Build history of the part. All positions in model axes, mm. A direction names the side the tool comes from. Give positions to 0.01 mm unless a question says otherwise; leave off trailing zeros. Order: outer loops, then holes, each group sorted by start corner. A loop starts at its lowest first (then second) coordinate and runs counter-clockwise, first axis right, second up. Notation, with made-up numbers: (-23.5, 73) -> (33.5, 73) arc R22 ccw to (33.5, 88) -> close; hole circle Ø9 at (3, -28). An arc over 180 degrees is marked (long way). One line per question, with ' | ' between items. Start each with the question number.
(1) Cut at A-A (y = 22). Give the cut face in (x, z), then the cut area to 3 significant figures.
(2) Pin check, flat tips, straight feed: pin 1 Ø5 at (x, y) = (-14, 23.5) entering from -Z; pin 2 Ø3 at (x, y) = (15, 23) entering from -Z; pin 3 Ø1.8 at (x, z) = (21, -28) entering from -Y. Stop position of each tip, or through.
(3) Cut at C-C (x = 20.5). Give the cut face in (y, z), then the cut area to 3 significant figures.
(4) Which spindle directions (+Z, -Z, +X, -X, +Y, -Y) get a long thin tool onto all of the face, cutting with end or side? Do faces 1 (the face through (0, 4, -21)), 2 (the face through (21.65, 0.99, -29.65)), 3 (the face through (-1, 7, -2)), 4 (the face through (0, 0, -20)), 5 (the face through (0, 15, -2)). Say none if no direction does.
(5) Cut at D-D (z = -22.5). Give the cut face in (x, y), then the cut area to 3 significant figures.
(6) Drill centre lines: L1, parallel to X at y = 22, z = -0.7; L2, parallel to X at y = 0.8, z = -26.88; L3, parallel to Z at x = -1.5, y = 33.5. Where is each one in solid material? Low to high. Write a range as from..to.
(7) Pull direction Z, two halves, no side cores. Call faces 6 (the face through (25, 3, -9)), 7 (the face through (0, 2, -37)), 8 (the face through (-14.26, 3.01, -27.04)), 9 (the face through (19.28, 3.01, -27.15)): +Z half, -Z half, draft (parallel to the pull), parting line (faces both ways), or undercut.
(8) Cut at B-B (z = -26.88). Give the cut face in (x, y), then the cut area to 3 significant figures.
from build123d import *

# Parameters (mm, degrees)
RESSALTO_EXTRUS_O1_DEPTH = 25
CORTE_EXTRUS_O1_START    = -4
ESBO_O2_R                = 3
ESBO_O2_R_2              = 1.25
CORTE_EXTRUS_O1_DEPTH    = 2
ESBO_O2_5_R              = 1.25
CORTE_EXTRUS_O2_DEPTH    = 58.358521599
ESBO_O2_6_R              = 1.25
CORTE_EXTRUS_O3_DEPTH    = 58.358521599
ESBO_O4_R                = 3
ESBO_O4_R_2              = 1.25
CORTE_EXTRUS_O4_DEPTH    = 2
ESBO_O4_4_R              = 1.25
CORTE_EXTRUS_O5_DEPTH    = 58.567351858
CORTE_EXTRUS_O8_START    = -4
CORTE_EXTRUS_O8_DEPTH    = 2
CORTE_EXTRUS_O9_DEPTH    = 58.567351858
FILETE1_R                = 15
FILETE2_R                = 7
FILETE3_R                = 0.25
FILETE4_R                = 3


with BuildPart() as part:
    # Esboço1 → Ressalto-extrusão1 (new, symmetric)
    with BuildSketch(Plane(origin=(0, 0, 0), x_dir=(0, 0, -1), z_dir=(1, 0, 0))):
        Polygon((0, 0), (37, 0), (37, 4), (4, 4), (4, 40), (0, 40), align=None)
    extrude(amount=RESSALTO_EXTRUS_O1_DEPTH, both=True)

    # Esboço2 → Corte-extrusão1 (cut)
    # profile 1 of 2: a face of its own
    with BuildSketch(Plane(origin=(0, 4, 0), x_dir=(1, 0, 0), z_dir=(0, 1, 0)).offset(CORTE_EXTRUS_O1_START)):
        with Locations(Location((20.5, 26.88, 0), (0, 0, 90))):
            Circle(ESBO_O2_R)
        with Locations(Location((20.5, 26.88, 0), (0, 0, 90))):
            Circle(ESBO_O2_R_2, mode=Mode.SUBTRACT)
    # profile 2 of 2: a face of its own
    with BuildSketch(Plane(origin=(0, 4, 0), x_dir=(1, 0, 0), z_dir=(0, 1, 0)).offset(CORTE_EXTRUS_O1_START)):
        with Locations(Location((-15.5, 26.88, 0), (0, 0, 90))):
            Circle(ESBO_O2_R)
        with Locations(Location((-15.5, 26.88, 0), (0, 0, 90))):
            Circle(ESBO_O2_R_2, mode=Mode.SUBTRACT)
    extrude(amount=CORTE_EXTRUS_O1_DEPTH, mode=Mode.SUBTRACT)

    # Esboço2<5> → Corte-extrusão2 (cut, through all)
    with BuildSketch(Plane(origin=(0, 4, 0), x_dir=(1, 0, 0), z_dir=(0, 1, 0))):
        with Locations(Location((-15.5, 26.88, 0), (0, 0, 270))):
            Circle(ESBO_O2_5_R)
    extrude(amount=-CORTE_EXTRUS_O2_DEPTH, mode=Mode.SUBTRACT)

    # Esboço2<6> → Corte-extrusão3 (cut, through all)
    with BuildSketch(Plane(origin=(0, 4, 0), x_dir=(1, 0, 0), z_dir=(0, 1, 0))):
        with Locations(Location((20.5, 26.88, 0), (0, 0, 270))):
            Circle(ESBO_O2_6_R)
    extrude(amount=-CORTE_EXTRUS_O3_DEPTH, mode=Mode.SUBTRACT)

    # Esboço4 → Corte-extrusão4 (cut)
    # profile 1 of 6: a face of its own
    with BuildSketch(Plane(origin=(0, 0, -4), x_dir=(-1, 0, 0), z_dir=(0, 0, -1))):
        with Locations(Location((14, 22, 0), (0, 0, 90))):
            Circle(ESBO_O4_R)
        with Locations(Location((14, 22, 0), (0, 0, 90))):
            Circle(ESBO_O4_R_2, mode=Mode.SUBTRACT)
    # profile 2 of 6: a face of its own
    with BuildSketch(Plane(origin=(0, 0, -4), x_dir=(-1, 0, 0), z_dir=(0, 0, -1))):
        with Locations(Location((-14, 22, 0), (0, 0, 90))):
            Circle(ESBO_O4_R)
        with Locations(Location((-14, 22, 0), (0, 0, 90))):
            Circle(ESBO_O4_R_2, mode=Mode.SUBTRACT)
    # profile 3 of 6: a face of its own
    with BuildSketch(Plane(origin=(0, 0, -4), x_dir=(-1, 0, 0), z_dir=(0, 0, -1))):
        with BuildLine():
            ThreePointArc((3, 8), (2.121320344, 10.121320344), (0, 11))
            Line((0, 11), (0, 9.25))
            ThreePointArc((0, 9.25), (0.883883476, 8.883883476), (1.25, 8))
            ThreePointArc((1.25, 8), (0.883883476, 7.116116524), (0, 6.75))
            Line((0, 6.75), (0, 5))
            ThreePointArc((0, 5), (2.121320344, 5.878679656), (3, 8))
        make_face()
    # profile 4 of 6: a face of its own
    with BuildSketch(Plane(origin=(0, 0, -4), x_dir=(-1, 0, 0), z_dir=(0, 0, -1))):
        with BuildLine():
            Line((0, 9.25), (0, 11))
            ThreePointArc((0, 11), (-3, 8), (0, 5))
            Line((0, 5), (0, 6.75))
            ThreePointArc((0, 6.75), (-1.25, 8), (0, 9.25))
        make_face()
    # profile 5 of 6: a face of its own
    with BuildSketch(Plane(origin=(0, 0, -4), x_dir=(-1, 0, 0), z_dir=(0, 0, -1))):
        with BuildLine():
            ThreePointArc((3, 8), (2.121320344, 10.121320344), (0, 11))
            Line((0, 11), (0, 9.25))
            ThreePointArc((0, 9.25), (0.883883476, 8.883883476), (1.25, 8))
            ThreePointArc((1.25, 8), (0.883883476, 7.116116524), (0, 6.75))
            Line((0, 6.75), (0, 5))
            ThreePointArc((0, 5), (2.121320344, 5.878679656), (3, 8))
        make_face()
    # profile 6 of 6: a face of its own
    with BuildSketch(Plane(origin=(0, 0, -4), x_dir=(-1, 0, 0), z_dir=(0, 0, -1))):
        with BuildLine():
            Line((0, 9.25), (0, 11))
            ThreePointArc((0, 11), (-3, 8), (0, 5))
            Line((0, 5), (0, 6.75))
            ThreePointArc((0, 6.75), (-1.25, 8), (0, 9.25))
        make_face()
    extrude(amount=-CORTE_EXTRUS_O4_DEPTH, mode=Mode.SUBTRACT)

    # Esboço4<4> → Corte-extrusão5 (cut, through all)
    with BuildSketch(Plane(origin=(0, 0, -4), x_dir=(-1, 0, 0), z_dir=(0, 0, -1))):
        with Locations(Location((-14, 22, 0), (0, 0, 90))):
            Circle(ESBO_O4_4_R)
        with Locations(Location((14, 22, 0), (0, 0, 90))):
            Circle(ESBO_O4_4_R)
        with BuildLine():
            ThreePointArc((1.25, 8), (0.883883476, 8.883883476), (0, 9.25))
            Line((0, 9.25), (0, 6.75))
            ThreePointArc((0, 6.75), (0.883883476, 7.116116524), (1.25, 8))
        make_face()
        with BuildLine():
            Line((0, 6.75), (0, 9.25))
            ThreePointArc((0, 9.25), (-1.25, 8), (0, 6.75))
        make_face()
    extrude(amount=-CORTE_EXTRUS_O5_DEPTH, mode=Mode.SUBTRACT)

    # Esboço4<11> → Corte-extrusão8 (cut)
    with BuildSketch(Plane(origin=(0, 0, -4), x_dir=(-1, 0, 0), z_dir=(0, 0, -1)).offset(CORTE_EXTRUS_O8_START)):
        with BuildLine():
            ThreePointArc((3, 16.65), (2.121320344, 18.771320344), (0, 19.65))
            Line((0, 19.65), (0, 17.9))
            ThreePointArc((0, 17.9), (0.883883476, 17.533883476), (1.25, 16.65))
            ThreePointArc((1.25, 16.65), (0.883883476, 15.766116524), (0, 15.4))
            Line((0, 15.4), (0, 13.65))
            ThreePointArc((0, 13.65), (2.121320344, 14.528679656), (3, 16.65))
        make_face()
        with BuildLine():
            Line((0, 17.9), (0, 19.65))
            ThreePointArc((0, 19.65), (-3, 16.65), (0, 13.65))
            Line((0, 13.65), (0, 15.4))
            ThreePointArc((0, 15.4), (-1.25, 16.65), (0, 17.9))
        make_face()
        with BuildLine():
            ThreePointArc((3, 35), (2.121320344, 37.121320344), (0, 38))
            Line((0, 38), (0, 36.25))
            ThreePointArc((0, 36.25), (0.883883476, 35.883883476), (1.25, 35))
            ThreePointArc((1.25, 35), (0.883883476, 34.116116524), (0, 33.75))
            Line((0, 33.75), (0, 32))
            ThreePointArc((0, 32), (2.121320344, 32.878679656), (3, 35))
        make_face()
        with BuildLine():
            Line((0, 36.25), (0, 38))
            ThreePointArc((0, 38), (-3, 35), (0, 32))
            Line((0, 32), (0, 33.75))
            ThreePointArc((0, 33.75), (-1.25, 35), (0, 36.25))
        make_face()
    extrude(amount=CORTE_EXTRUS_O8_DEPTH, mode=Mode.SUBTRACT)

    # Esboço4<12> → Corte-extrusão9 (cut, through all)
    with BuildSketch(Plane(origin=(0, 0, -4), x_dir=(-1, 0, 0), z_dir=(0, 0, -1))):
        with BuildLine():
            ThreePointArc((1.25, 35), (0.883883476, 35.883883476), (0, 36.25))
            Line((0, 36.25), (0, 33.75))
            ThreePointArc((0, 33.75), (0.883883476, 34.116116524), (1.25, 35))
        make_face()
        with BuildLine():
            Line((0, 33.75), (0, 36.25))
            ThreePointArc((0, 36.25), (-1.25, 35), (0, 33.75))
        make_face()
        with BuildLine():
            ThreePointArc((1.25, 16.65), (0.883883476, 17.533883476), (0, 17.9))
            Line((0, 17.9), (0, 15.4))
            ThreePointArc((0, 15.4), (0.883883476, 15.766116524), (1.25, 16.65))
        make_face()
        with BuildLine():
            Line((0, 15.4), (0, 17.9))
            ThreePointArc((0, 17.9), (-1.25, 16.65), (0, 15.4))
        make_face()
    extrude(amount=-CORTE_EXTRUS_O9_DEPTH, mode=Mode.SUBTRACT)

    # Filete1
    filete1_edges = [part.edges().sort_by_distance(p)[0] for p in [
        (25, 40, -2),
        (-25, 40, -2),
    ]]
    fillet(filete1_edges, radius=FILETE1_R)

    # Filete2
    filete2_edges = [part.edges().sort_by_distance(p)[0] for p in [
        (25, 2, -37),
        (-25, 2, -37),
    ]]
    fillet(filete2_edges, radius=FILETE2_R)

    # Filete3
    filete3_edges = [part.edges().sort_by_distance(p)[0] for p in [
        (0, 4, -4),
    ]]
    fillet(filete3_edges, radius=FILETE3_R)

    # Filete4
    filete4_edges = [part.edges().sort_by_distance(p)[0] for p in [
        (0, 0, 0),
    ]]
    fillet(filete4_edges, radius=FILETE4_R)


solid = part.part
Result set:
1) outline: (-25, -4) -> (-17, -4) -> (-17, -2) -> (-15.25, -2) -> (-15.25, 0) -> (-25, 0) -> close; (-12.75, -2) -> (-11, -2) -> (-11, -4) -> (11, -4) -> (11, -2) -> (12.75, -2) -> (12.75, 0) -> (-12.75, 0) -> close; (15.25, -2) -> (17, -2) -> (17, -4) -> (25, -4) -> (25, 0) -> (15.25, 0) -> close | area: 166 mm2
2) pin 1: stops at z = -4 | pin 2: stops at z = -2 | pin 3: stops at y = 2
3) outline: (0, -36.54) -> (4, -36.54) -> (4, -28.13) -> (2, -28.13) -> (2, -29.88) -> (0, -29.88) -> close; (0, -23.88) -> (2, -23.88) -> (2, -25.63) -> (4, -25.63) -> (4, -4.25) arc R0.25 cw to (4.25, -4) -> (35.71, -4) -> (35.71, 0) -> (3, 0) arc R3 ccw to (0, -3) -> close | area: 254 mm2
4) face 1: -Z, +X, -X, +Y | face 2: -Y | face 3: -Z | face 4: +Z, -Z, +X, -X, -Y | face 5: +Z
5) outline: (-25, 0) -> (25, 0) -> (25, 4) -> (-25, 4) -> close | area: 200 mm2
6) L1: x = -25..-15.25, -12.75..12.75, 15.25..25 | L2: x = -25..-18.5, -12.5..17.5, 23.5..25 | L3: z = -4..-2
7) face 6: draft | face 7: -Z half | face 8: undercut | face 9: undercut
8) outline: (-25, 0) -> (-18.5, 0) -> (-18.5, 2) -> (-16.75, 2) -> (-16.75, 4) -> (-25, 4) -> close; (-14.25, 2) -> (-12.5, 2) -> (-12.5, 0) -> (17.5, 0) -> (17.5, 2) -> (19.25, 2) -> (19.25, 4) -> (-14.25, 4) -> close; (21.75, 2) -> (23.5, 2) -> (23.5, 0) -> (25, 0) -> (25, 4) -> (21.75, 4) -> close | area: 166 mm2
